Here's the drawing with two shaded views (mm, measured from the low corner). I have some questions. A direction names the side the tool comes from. Round coordinates to 2 decimals unless told otherwise and drop trailing zeros. Loops run counter-clockwise (first coordinate to the right, second up) from the corner with the lowest first, then second, coordinate; pieces in that order, holes last.
(1) I want a section at B-B on z = 55. Write out the boundary of the cut face in (x, y), plus the area to 3 significant figures.
(2) Will these pins go through, and if not, where does the flat tip stop? pin 1 Ø8 at (x, z) = (255.5, 76) entering from +Y; pin 2 Ø4 at (y, z) = (73, 31.2) entering from +X; pin 3 Ø4 at (y, z) = (73, 46.2) entering from -X.
(3) I want a section at A-A on y = 54.5. Write out the boundary of the cut face in (x, z).
(4) Thinking about a two-plate mould opening in X: for the marked faces 3, 4 and 5, which applies, released by +X, released by -X, zero draft, split by the parting line, or undercut?
(5) I want a section at C-C on x = 253. Write out the boundary of the cut face in (y, z), plus the area to 3 significant figures.
(6) If I drill on line 1 along X through (y, z) = (8, 71.5); line 2 along Y through (x, z) = (217, 25.5); line 3 along X through (y, z) = (71, 16), over which ranges is the centre line in solid material (lowest first)?
(7) Which directions (+Z, -Z, +X, -X, +Y, -Y) give clear straight access to the entire face, cutting with the end or side of a thin tool? Please do the marked faces 1 and 2.
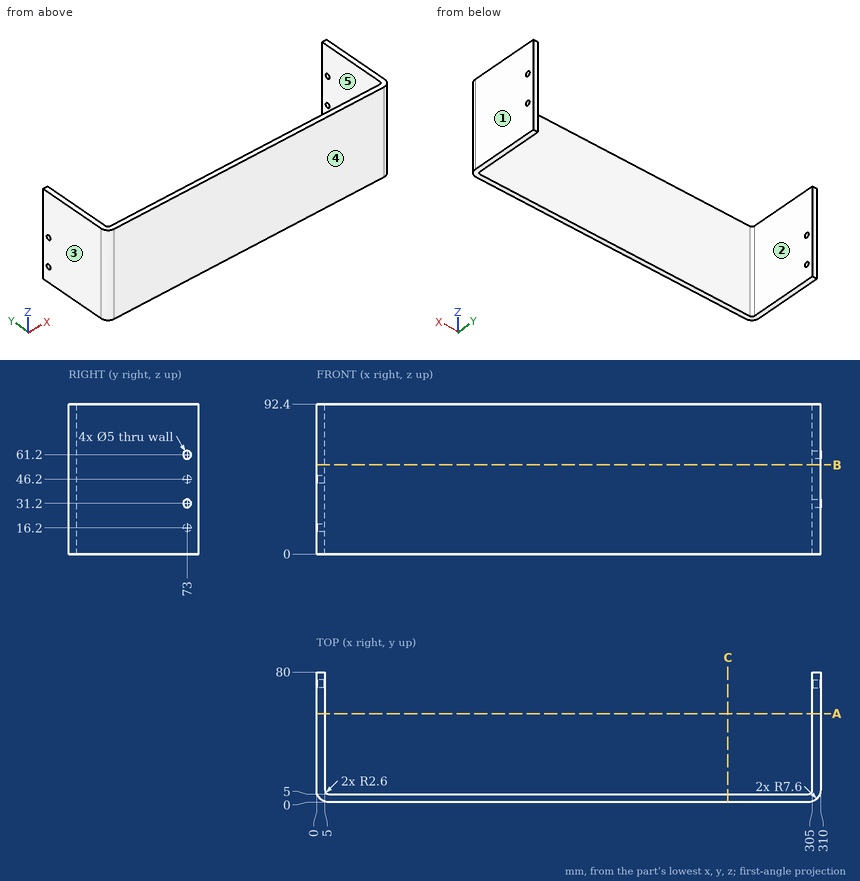
Filled sheet:
1. outline: (0, 7.6) arc R7.6 ccw to (7.6, 0) - (302.4, 0) arc R7.6 ccw to (310, 7.6) - (310, 80) - (305, 80) - (305, 7.6) arc R2.6 cw to (302.4, 5) - (7.6, 5) arc R2.6 cw to (5, 7.6) - (5, 80) - (0, 80) - close
1. area: 2,280 mm2
2. pin 1: stops at y = 5
2. pin 2: stops at x = 5
2. pin 3: stops at x = 305
3. outline: (0, 0) - (5, 0) - (5, 92.4) - (0, 92.4) - close; (305, 0) - (310, 0) - (310, 92.4) - (305, 92.4) - close
4. face 3: released by -X
4. face 4: zero draft
4. face 5: undercut
5. outline: (0, 0) - (5, 0) - (5, 92.4) - (0, 92.4) - close
5. area: 462 mm2
6. line 1: x = 0 to 5, 305 to 310
6. line 2: y = 0 to 5
6. line 3: x = 305 to 310
7. face 1: +Z, -Z, +X, +Y, -Y
7. face 2: +Z, -Z, +Y
